```python
from build123d import *

# Parameters (mm, degrees)
BOSS_EXTRU_1_DEPTH                                 = 22
ESQUISSE2_W                                        = 22
ESQUISSE2_H                                        = 6
BOSS_EXTRU_2_DEPTH                                 = 5
CHAMBRAGE_POUR_VIS_T_TE_HEXAGONALE_M21_D           = 2.4
CHAMBRAGE_POUR_VIS_T_TE_HEXAGONALE_M21_CBORE_D     = 4.4
CHAMBRAGE_POUR_VIS_T_TE_HEXAGONALE_M21_CBORE_DEPTH = 2.4
CONG_1_R                                           = 10
CONG_2_R                                           = 1


with BuildPart() as part:
    # Esquisse1 → Boss.-Extru.1 (new body)
    with BuildSketch(Plane.XY):
        with BuildLine():
            Line((0, 6), (0, 0))
            Line((0, 0), (6, 0))
            ThreePointArc((6, 0), (11, 5), (16, 0))
            Line((16, 0), (22, 0))
            Line((22, 0), (22, 6))
            Line((22, 6), (0, 6))
        make_face()
    extrude(amount=BOSS_EXTRU_1_DEPTH)

    # Esquisse2 → Boss.-Extru.2 (add)
    with BuildSketch(Plane.XY.offset(22)):
        with Locations((11, 3)):
            Rectangle(ESQUISSE2_W, ESQUISSE2_H)
    extrude(amount=BOSS_EXTRU_2_DEPTH)

    # Chambrage pour vis à tête hexagonale M21 (through all)
    with Locations(Plane(origin=(0, 6, 0), x_dir=(1, 0, 0), z_dir=(0, 1, 0))):
        with Locations((19, -12), (3, -12)):
            CounterBoreHole(CHAMBRAGE_POUR_VIS_T_TE_HEXAGONALE_M21_D / 2, CHAMBRAGE_POUR_VIS_T_TE_HEXAGONALE_M21_CBORE_D / 2, CHAMBRAGE_POUR_VIS_T_TE_HEXAGONALE_M21_CBORE_DEPTH)

    # Congé1
    # the kernel refuses this fillet: 10 mm, written as the material it takes off along each edge
    with BuildSketch(Plane(origin=(0, 31, 0), x_dir=(0, 0, 1), z_dir=(0, -1, 0)), Plane(origin=(22, -25, 27), x_dir=(-1, 0, 0), z_dir=(0, 1, 0))) as cong_1_piece_1:
        with BuildLine():
            CenterArc((CONG_1_R, -CONG_1_R), CONG_1_R, 90, 90)
            Line((0, -CONG_1_R), (0, 0))
            Line((0, 0), (CONG_1_R, 0))
        make_face()
    extrude(amount=56, mode=Mode.SUBTRACT)
    with BuildSketch(Plane(origin=(0, 31, 27), x_dir=(0, 0, -1), z_dir=(0, -1, 0)), Plane(origin=(22, -25, 0), x_dir=(-1, 0, 0), z_dir=(0, 1, 0))) as cong_1_piece_2:
        with BuildLine():
            CenterArc((CONG_1_R, CONG_1_R), CONG_1_R, 180, 90)
            Line((0, CONG_1_R), (0, 0))
            Line((0, 0), (CONG_1_R, 0))
        make_face()
    extrude(amount=56, mode=Mode.SUBTRACT)

    # Congé2
    # the kernel refuses this fillet: 1 mm, written as the material it takes off along each edge
    with BuildSketch(Plane(origin=(12, 6, 0), x_dir=(0, 0, 1), z_dir=(-1, 0, 0))) as cong_2_piece_1:
        with BuildLine():
            CenterArc((CONG_2_R, -CONG_2_R), CONG_2_R, 90, 90)
            Line((0, -CONG_2_R), (0, 0))
            Line((0, 0), (CONG_2_R, 0))
        make_face()
    extrude(amount=2, mode=Mode.SUBTRACT)
    with BuildSketch(Plane(origin=(0, 6, 17), x_dir=(0, -1, 0), z_dir=(0, 0, -1)), Plane(origin=(22, 6, 17), x_dir=(-1, 0, 0), z_dir=(0, 0, -1))) as cong_2_piece_2:
        with BuildLine():
            CenterArc((CONG_2_R, -CONG_2_R), CONG_2_R, 90, 90)
            Line((0, -CONG_2_R), (0, 0))
            Line((0, 0), (CONG_2_R, 0))
        make_face()
    extrude(amount=7, mode=Mode.SUBTRACT)
    with BuildSketch(Plane(origin=(12, 6, 27), x_dir=(0, 0, -1), z_dir=(-1, 0, 0))) as cong_2_piece_3:
        with BuildLine():
            CenterArc((CONG_2_R, CONG_2_R), CONG_2_R, 180, 90)
            Line((0, CONG_2_R), (0, 0))
            Line((0, 0), (CONG_2_R, 0))
        make_face()
    extrude(amount=2, mode=Mode.SUBTRACT)
    with BuildSketch(Plane(origin=(12, 6, 17), x_dir=(1, 0, 0), z_dir=(0, 0, -1))) as cong_2_piece_4:
        with BuildLine():
            CenterArc((10 - CONG_2_R, CONG_2_R), CONG_2_R, 270, 90)
            Line((10, CONG_2_R), (10, 0))
            Line((10, 0), (10 - CONG_2_R, 0))
        make_face()
    revolve(axis=Axis((12, 6, 17), (0, -1, 0)), revolution_arc=90, mode=Mode.SUBTRACT)
    with BuildSketch(Plane(origin=(12, 6, 10), x_dir=(0, 0, -1), z_dir=(-1, 0, 0))) as cong_2_piece_5:
        with BuildLine():
            CenterArc((10 - CONG_2_R, CONG_2_R), CONG_2_R, 270, 90)
            Line((10, CONG_2_R), (10, 0))
            Line((10, 0), (10 - CONG_2_R, 0))
        make_face()
    revolve(axis=Axis((12, 6, 10), (0, -1, 0)), revolution_arc=90, mode=Mode.SUBTRACT)
    with BuildSketch(Plane(origin=(10, 6, 17), x_dir=(-1, 0, 0), z_dir=(0, 0, -1))) as cong_2_piece_6:
        with BuildLine():
            CenterArc((10 - CONG_2_R, -CONG_2_R), CONG_2_R, 0, 90)
            Line((10, -CONG_2_R), (10, 0))
            Line((10, 0), (10 - CONG_2_R, 0))
        make_face()
    revolve(axis=Axis((10, 6, 17), (0, 1, 0)), revolution_arc=90, mode=Mode.SUBTRACT)
    with BuildSketch(Plane(origin=(10, 6, 10), x_dir=(0, 0, -1), z_dir=(1, 0, 0))) as cong_2_piece_7:
        with BuildLine():
            CenterArc((10 - CONG_2_R, -CONG_2_R), CONG_2_R, 0, 90)
            Line((10, -CONG_2_R), (10, 0))
            Line((10, 0), (10 - CONG_2_R, 0))
        make_face()
    revolve(axis=Axis((10, 6, 10), (0, 1, 0)), revolution_arc=90, mode=Mode.SUBTRACT)


solid = part.part
```
Design review of the part built by this model. Coordinates are the model's own, in mm. A direction names the side the tool comes from. Coordinates: 2 decimals unless noted, no trailing zeros. Write each loop counter-clockwise with the first axis right and the second up, starting at its lowest first coordinate (ties: lowest second). Pieces come first, ordered by that corner, then holes.
1) Add section A-A (z = 14.75). Write out the cut boundary in (x, y), plus the area to 3 significant figures.
2) Machinability: for faces 4 (the flat face through (11, 6, 13)), 5 (the cylindrical face through (1.38, 4.82, 10.51)), 6 (the flat face through (11, 2, 22)), which of the approach directions +Z, -Z, +X, -X, +Y, -Y give a long, thin tool a straight path to every point of the face, cutting with its end or side? Answer none if there is none.
3) Add section B-B (y = 2.25). Write out the cut boundary in (x, z).
4) Add section C-C (y = 5.5). Write out the cut boundary in (x, z), plus the area to 3 significant figures.
5) To check wall thickness, follow L1, parallel to X at y = 5.3, z = 12; L2, parallel to X at y = 0.8, z = 12; L3, parallel to X at y = 1.4, z = 12. State the ranges of each line that lie inside material, in increasing order.
6) Insertion check: pin 1 (2 mm diameter, centred on x = 3, z = 12, fed in from -Y); pin 2 (1 mm diameter, centred on x = 19, y = 1, fed in from -Z); pin 3 (2 mm diameter, centred on x = 15.5, y = 1.5, fed in from -Z); pin 4 (3.5 mm diameter, centred on x = 3, z = 12, fed in from +Y). Each pin has a flat end and moves straight along its axis. Give the tip position at first contact, or say it passes through.
7) Add section D-D (y = 0.5). Write out the cut boundary in (x, z), plus the area to 3 significant figures.
8) Mouldability with a two-part tool opening along Z and no side actions: class faces 1 (the cylindrical face through (20, 2, 4)), 2 (the flat face through (11, 3, 27)), 3 (the flat face through (20, 3.6, 13)) as +Z half, -Z half, draft (parallel to the pull), parting line (faces both ways), or undercut.
Check result:
1. outline: (0, 0) - (6, 0) arc R5 cw to (16, 0) - (22, 0) - (22, 5) arc R1 ccw to (21, 6) - (1, 6) arc R1 ccw to (0, 5) - close
1. area: 92.3 mm2
2. face 4: +Z, -Z, +X, -X, +Y
2. face 5: +Y
2. face 6: -Z, -Y
3. outline: (0, 10) arc R10 ccw to (6.53, 0.62) - (6.53, 22) - (15.47, 22) - (15.47, 0.62) arc R10 ccw to (22, 10) - (22, 17) arc R10 ccw to (12, 27) - (10, 27) arc R10 ccw to (0, 17) - close; hole circle Ø2.4 at (3, 12); hole circle Ø2.4 at (19, 12)
4. outline: (0.13, 10) arc R9.87 ccw to (10, 0.13) - (12, 0.13) arc R9.87 ccw to (21.87, 10) - (21.87, 17) arc R9.87 ccw to (12, 26.87) - (10, 26.87) arc R9.87 ccw to (0.13, 17) - close; hole circle Ø4.4 at (3, 12); hole circle Ø4.4 at (19, 12)
4. area: 467 mm2
5. L1: x = 0.05 to 0.8, 5.2 to 16.8, 21.2 to 21.95
5. L2: x = 0 to 1.8, 4.2 to 6.06, 15.94 to 17.8, 20.2 to 22
5. L3: x = 0 to 1.8, 4.2 to 6.2, 15.8 to 17.8, 20.2 to 22
6. pin 1: passes through
6. pin 2: stops at z = 2.4
6. pin 3: stops at z = 0.57
6. pin 4: stops at y = 3.6
7. outline: (0, 10) arc R10 ccw to (6.03, 0.82) - (6.03, 22) - (15.97, 22) - (15.97, 0.82) arc R10 ccw to (22, 10) - (22, 17) arc R10 ccw to (12, 27) - (10, 27) arc R10 ccw to (0, 17) - close; hole circle Ø2.4 at (3, 12); hole circle Ø2.4 at (19, 12)
7. area: 282 mm2
8. face 1: -Z half
8. face 2: +Z half
8. face 3: undercut
